from build123d import *

# Parameters (mm, degrees)
F_12_CLEARANCE_HOLE1_D = 5.7912
CIRPATTERN1_COUNT      = 4


with BuildPart() as part:
    # Sketch1 → Revolve1 (revolve)
    with BuildSketch(Plane.XY):
        with BuildLine():
            Line((4.7625, 12.547042688), (4.7625, 17.143351136))
            Line((4.7625, 17.143351136), (20.20283565, 17.143351136))
            Line((20.20283565, 17.143351136), (20.20283565, 22.067968078))
            Line((20.20283565, 22.067968078), (49.112399892, 22.067968078))
            Line((49.112399892, 22.067968078), (49.112399892, 23.05289127))
            Line((49.112399892, 23.05289127), (54.368684681, 23.05289127))
            Line((54.368684681, 23.05289127), (54.368684681, 25.4))
            Line((54.368684681, 25.4), (7.14375, 25.4))
            ThreePointArc((7.14375, 25.4), (5.459951977, 26.097451977), (4.7625, 27.78125))
            Line((4.7625, 27.78125), (4.7625, 50.00625))
            Line((4.7625, 50.00625), (3.96875, 50.8))
            Line((3.96875, 50.8), (0.79375, 50.8))
            Line((0.79375, 50.8), (0, 50.00625))
            Line((0, 50.00625), (0, 17.143351136))
            Line((0, 17.143351136), (4.7625, 12.547042688))
        make_face()
    revolve(axis=Axis((207.498884421, 0, 0), (1, 0, 0)))

    # #12 Clearance Hole1 (through all)
    with Locations(Plane(origin=(0, 33.069002249, -0.146973343), x_dir=(0, 0, -1), z_dir=(-1, 0, 0))):
        with Locations((0, 0)):
            f_12_clearance_hole1 = Hole(F_12_CLEARANCE_HOLE1_D / 2)

    # CirPattern1: #12 Clearance Hole1 ×4 about axis
    cirpattern1_axis = Axis((0, 0, 0), (1, 0, 0))
    for i in range(1, CIRPATTERN1_COUNT):
        add(f_12_clearance_hole1.rotate(cirpattern1_axis, i * 360 / CIRPATTERN1_COUNT), mode=Mode.SUBTRACT)


solid = part.part
Input: part model. Units: mm. Frame: model coordinates. A direction names the side the tool comes from. Round coordinates to 2 decimals unless told otherwise and drop trailing zeros. Order: outer loops, then holes, each group sorted by start corner. A loop starts at its lowest first (then second) coordinate and runs counter-clockwise, first axis right, second up. Notation, with made-up numbers: (43.5, -10.5) - (58.5, -10.5) arc R32 cw to (58.5, 16.5) - close; hole circle Ø3 at (58.25, -36). An arc over 180 degrees is marked (long way). Answer as a JSON object with one key per item and string values. Group by question number.
(1) Material intervals for probe 1 along Y at (x, z) = (24.5, -0.5); probe 2 along Z at (x, y) = (14, 0); probe 3 along X at (y, z) = (29, -26.5), sorted ascending. Write a range as from..to.
(2) Cut plane D-D (x = 16). Return loops of the section in (y, z), then the cut area to 3 significant figures.
(3) Draft query along Y for faces 3 (the face through (2.415, -0.775, -35.896)), 4 (the face through (54.369, 5.8, -22.5)), 5 (the face through (2.359, -11.012, -49.592)). Return one class per face: released by +Y, released by -Y, zero draft, split by the parting line, or undercut.
(4) Cut plane A-A (x = 25). Return loops of the section in (y, z), then the cut area to 3 significant figures.
(5) Pin query (flat end, axial travel): P1, Ø23, axis at y = -7, z = -6, coming from the +X side; P2, Ø1.5, axis at x = 32, y = 23, coming from the +Z side; P3, Ø5, axis at x = 36, z = 11.5, coming from the -Y side. Return the tip coordinate at first contact, or that it passes through.
(6) Reachability of faces 1 (the face through (2.415, -1.189, 35.638)), 2 (the face through (30.426, -5.506, -24.796)) from +Z, -Z, +X, -X, +Y, -Y: full face, straight path, thin tool, end or side. Return the list, or none.
(7) Cut plane B-B (y = 0). Count the separate pieces of the cut face and the enclosed holes in it, then the cut area to 3 significant figures.
Here are the results:
{
 "1": {"probe 1": "y = -25.4..-22.06, 22.06..25.4", "probe 2": "z = -25.4..-17.14, 17.14..25.4", "probe 3": "x = 0..4.76"},
 "2": {"outline": "circle Ø50.8 at (0, 0); hole circle Ø34.29 at (0, 0)", "area": "1,100 mm^2"},
 "3": {"face 3": "undercut", "face 4": "zero draft", "face 5": "split by the parting line"},
 "4": {"outline": "circle Ø50.8 at (0, 0); hole circle Ø44.14 at (0, 0)", "area": "497 mm^2"},
 "5": {"P1": "stops at x = 20.2", "P2": "stops at z = 12.25", "P3": "stops at y = -23.75"},
 "6": {"face 1": "+X, -X", "face 2": "+X"},
 "7": {"separate pieces": "4", "enclosed holes": "0", "area": "761 mm^2"}
}
